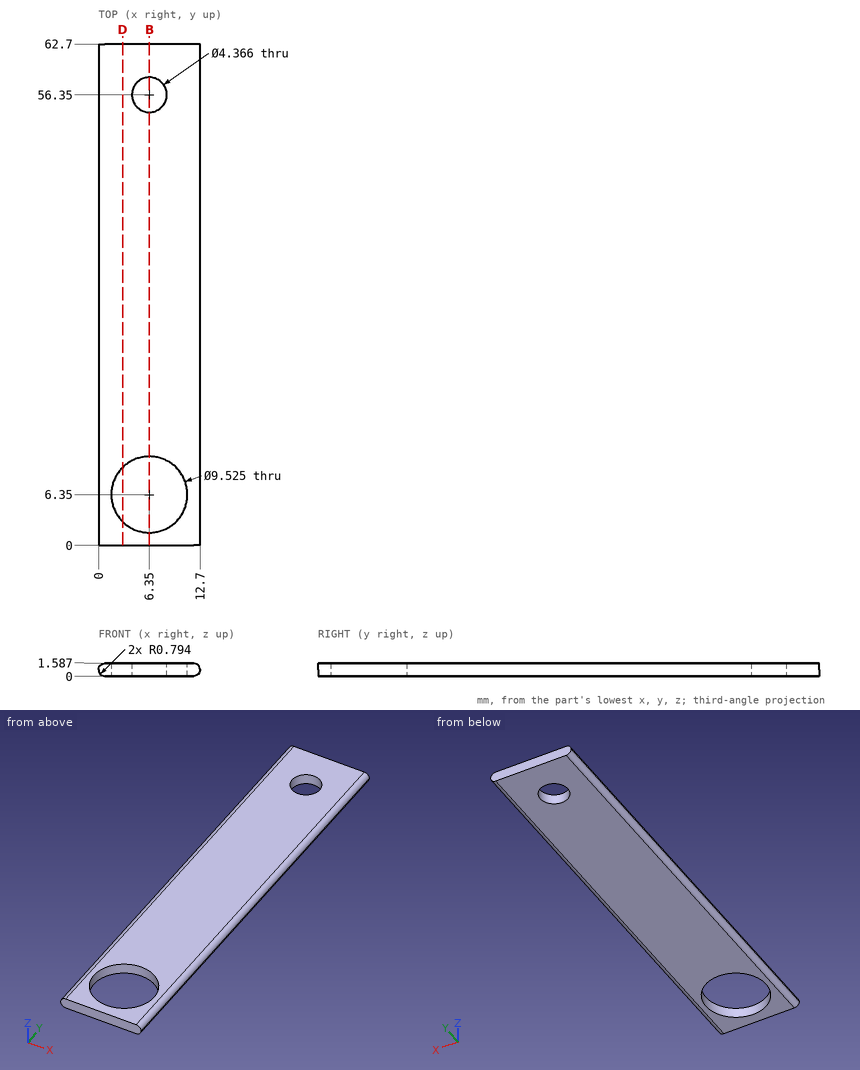
Geometry check sheet. Reference: drawing and pictorial views, mm from the part's lowest x, y, z. Give positions to 0.01 mm unless a question says otherwise; leave off trailing zeros. Order: outer loops, then holes, each group sorted by start corner. A loop starts at its lowest first (then second) coordinate and runs counter-clockwise, first axis right, second up.
1. Gauge pin test, flat end, axial feed: pin 1 Ø7 at (x, y) = (6.35, 56.35) entering from -Z. Record the tip position at first contact, or that the pin passes through.
2. Section check B-B, the plane x = 6.35. Enter the section's corners in (y, z).
3. Thickness scan on L1, parallel to Y at x = 6.35, z = 0.65; L2, parallel to Y at x = 10.25, z = 0.6 (1 decimal); L3, parallel to Y at x = 8.75, z = 0.3 (1 decimal). Record the ranges inside material, lowest first.
4. Section check D-D, the plane x = 3. Enter the section's corners in (y, z) (1 decimal).
Values follow:
1. pin 1: stops at z = 0
2. outline: (0, 0) - (1.59, 0) - (1.59, 1.59) - (0, 1.59) - close; (11.11, 0) - (54.17, 0) - (54.17, 1.59) - (11.11, 1.59) - close; (58.53, 0) - (62.7, 0) - (62.7, 1.59) - (58.53, 1.59) - close
3. L1: y = 0 to 1.59, 11.11 to 54.17, 58.53 to 62.7
3. L2: y = 0 to 3.6, 9.1 to 62.7
3. L3: y = 0 to 2.2, 10.5 to 62.7
4. outline: (0, 0) - (3, 0) - (3, 1.6) - (0, 1.6) - close; (9.7, 0) - (62.7, 0) - (62.7, 1.6) - (9.7, 1.6) - close
